from build123d import *

# Parameters (mm, degrees)
F0_R     = 12.5
F1_DEPTH = 25
F2_W     = 11
F2_H     = 23
F4_W     = 82.212326
F4_H     = 18.054354
F5_DEPTH = 52.001


with BuildPart() as f1:
    # F0 (on Top) → F1 (new body)
    with BuildSketch(Plane.XY):
        with BuildLine():
            ThreePointArc((0, 17.5), (5.125631, 5.125631), (17.5, 0))
            Line((17.5, 0), (62, 0))
            ThreePointArc((62, 0), (65.535534, 1.464466), (67, 5))
            Line((67, 5), (67, 47))
            ThreePointArc((67, 47), (65.535534, 50.535534), (62, 52))
            Line((62, 52), (5, 52))
            ThreePointArc((5, 52), (1.464466, 50.535534), (0, 47))
            Line((0, 47), (0, 17.5))
        make_face()
        with Locations((17.5, 17.5)):
            Circle(F0_R, mode=Mode.SUBTRACT)
    extrude(amount=F1_DEPTH)

    # F2 (on face) → F3 (revolve, cut)
    with BuildSketch(Plane.XY.offset(25)):
        with Locations((40.5, 14.5)):
            Rectangle(F2_W, F2_H)
        with Locations((56.5, 14.5)):
            Rectangle(F2_W, F2_H)
    revolve(axis=Axis((40.5, 26, 25), (1, 0, 0)), mode=Mode.SUBTRACT)

    # F4 (on face) → F5 (cut, through all)
    with BuildSketch(Plane.XZ):
        with Locations((41.106163, 27.027177)):
            Rectangle(F4_W, F4_H)
    extrude(amount=-F5_DEPTH, mode=Mode.SUBTRACT)


solid = f1.part
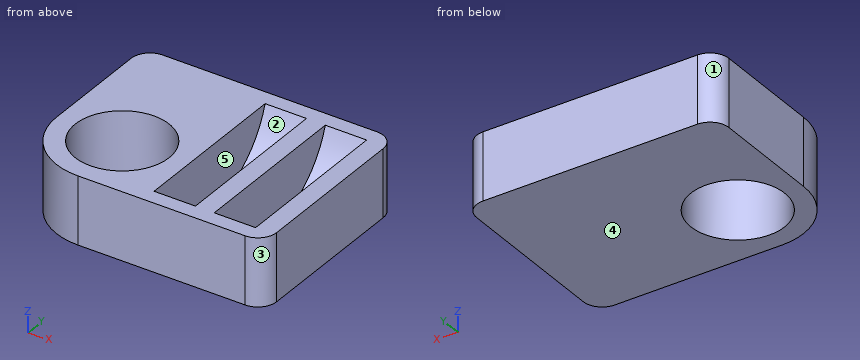
Can you work these out from the model? Positions are in its coordinate system, mm. Face numbers are marked on the shaded views. A direction names the side the tool comes from. Give positions to 0.01 mm unless a question says otherwise; leave off trailing zeros. Order: outer loops, then holes, each group sorted by start corner. A loop starts at its lowest first (then second) coordinate and runs counter-clockwise, first axis right, second up. Notation, with made-up numbers: M -30,-15 L 4,-15 A18 cw 4,20 Z; hole C -11.5,30 d8. An arc over 180 degrees is marked long. Use a Markdown table: item, result. Add a question column.
Item 1: Will these pins go through, and if not, where does the flat tip stop? pin 1 (20 mm diameter, centred on x = 17.5, y = 17.5, fed in from +Z); pin 2 (10 mm diameter, centred on x = 9, z = 9.5, fed in from -Y).
Item 2: We'd pull the mould along X, two halves only. Please class the marked faces 3, 4 and 5: +X half, -X half, draft (parallel to the pull), parting line (faces both ways), or undercut.
Item 3: For the marked faces 1 and 2, which set-ups out of +Z, -Z, +X, -X, +Y, -Y let a thin tool reach every point of the face, with its end or its side?
Item 4: Suppose I cut it at B-B (z = 13). List the corners of the cut face in (x, y) for me.
Item 5: If I drill on L1, parallel to X at y = 17.5, z = 14; L2, parallel to X at y = 42, z = 13.5; L3, parallel to Y at x = 17.5, z = 11.75, over which ranges is the centre line in solid material (lowest first)? Write a range as [from, to].
Item 6: Suppose I cut it at C-C (x = 52.5). List the corners of the cut face in (y, z) for me, then the cut area to 3 significant figures.
Item 7: Suppose I cut it at D-D (y = 43). List the corners of the cut face in (x, z) for me, then the cut area to 3 significant figures.
Item 8: Suppose I cut it at A-A (x = 11). List the corners of the cut face in (y, z) for me, then the cut area to 3 significant figures.
Answer sheet:
| question | item | result |
|---|---|---|
| 1 | pin 1 | passes through |
| 1 | pin 2 | stops at y = 0.35 |
| 2 | face 3 | +X half |
| 2 | face 4 | draft |
| 2 | face 5 | undercut |
| 3 | face 1 | +Z, -Z, -X, +Y |
| 3 | face 2 | +Z |
| 4 | outline | M 0,17.5 A17.5 ccw 17.5,0 L 62,0 A5 ccw 67,5 L 67,47 A5 ccw 62,52 L 5,52 A5 ccw 0,47 Z; hole C 17.5,17.5 d25; hole M 35,6.38 L 46,6.38 L 46,45.62 L 35,45.62 Z; hole M 51,6.38 L 62,6.38 L 62,45.62 L 51,45.62 Z |
| 5 | L1 | x = [0, 5], [30, 35], [46, 51], [62, 67] |
| 5 | L2 | x = [0, 35], [46, 51], [62, 67] |
| 5 | L3 | y = [0, 5], [30, 52] |
| 6 | outline | M 0,0 L 52,0 L 52,18 L 47.91,18 A23 cw 4.09,18 L 0,18 Z |
| 6 | area | 422 mm² |
| 7 | outline | M 0,0 L 67,0 L 67,18 L 62,18 L 62,9.51 L 51,9.51 L 51,18 L 46,18 L 46,9.51 L 35,9.51 L 35,18 L 0,18 Z |
| 7 | area | 1,020 mm² |
| 8 | outline | M 1.25,0 L 6.82,0 L 6.82,18 L 1.25,18 Z; M 28.18,0 L 52,0 L 52,18 L 28.18,18 Z |
| 8 | area | 529 mm² |
